Part print with two shaded views. Sizes in mm from the minimum x, y, z corner. Coordinates: 2 decimals unless noted, no trailing zeros. Loops run counter-clockwise (first coordinate to the right, second up) from the corner with the lowest first, then second, coordinate; pieces in that order, holes last. Notation, with made-up numbers: (49, 29) -> (97, 29) arc R22 cw to (97, 52) -> close; hole circle Ø1 at (71, 9.25). An arc over 180 degrees is marked (long way). Use one line per item in the form item = value.
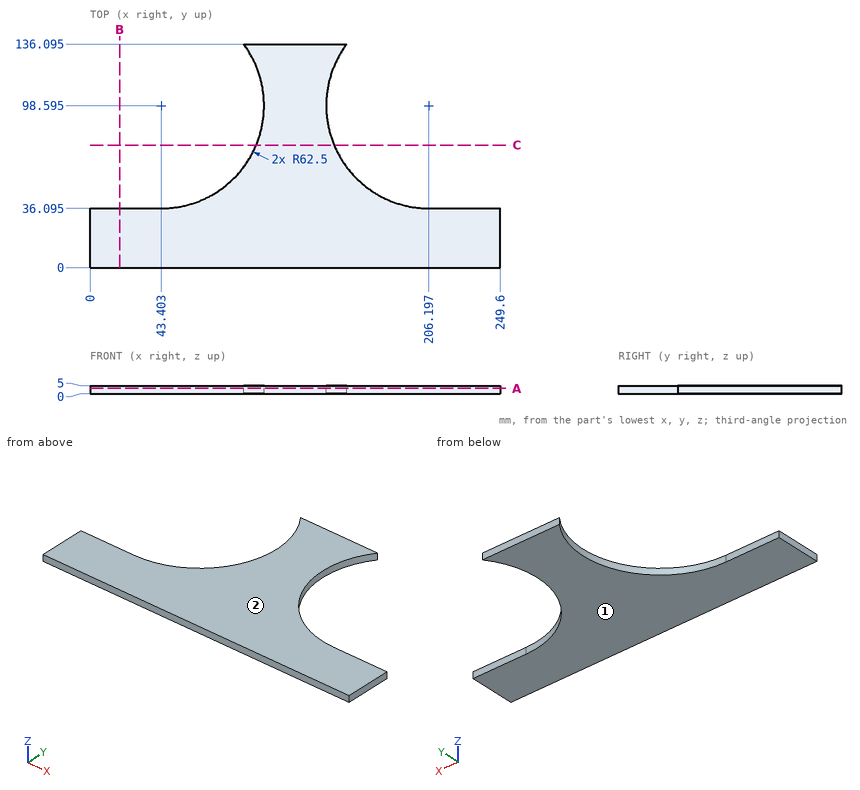
Q1. Band-saw the part on A-A, the plane z = 3.4. Write the cut outline in (x, y) (1 decimal).
Result:
outline = (0, 0) -> (249.6, 0) -> (249.6, 36.1) -> (206.2, 36.1) arc R62.5 cw to (156.2, 136.1) -> (93.4, 136.1) arc R62.5 cw to (43.4, 36.1) -> (0, 36.1) -> close
Q2. Band-saw the part on B-B, the plane x = 18. Write the cut outline in (y, z) (1 decimal).
Result:
outline = (0, 0) -> (36.1, 0) -> (36.1, 5) -> (0, 5) -> close
Q3. Mould opens along Z. For the marked faces 1 and 2 say: released by +Z, released by -Z, zero draft, split by the parting line, or undercut.
Result:
face_1 = released by -Z
face_2 = released by +Z
Q4. Wall check: line 1 along X through (y, z) = (100, 2.2); line 2 along Y through (x, z) = (17, 1.85) (1 decimal); line 3 along Y through (x, z) = (193, 0.2) (1 decimal). Give the ranges that are in metal, low to high.
Result:
line_1 = 105.89 to 143.71
line_2 = 0 to 36.1
line_3 = 0 to 37.5
Q5. Band-saw the part on C-C, the plane y = 74.5. Write the cut outline in (x, z), and give its area (3 significant figures).
Result:
outline = (101.07, 0) -> (148.53, 0) -> (148.53, 5) -> (101.07, 5) -> close
area = 237 mm2
Q6. Pin check, flat tips, straight feed: pin 1 Ø1 at (y, z) = (57.5, 1.5) entering from -X; pin 2 Ø1.5 at (x, z) = (224.5, 1.5) entering from +Y (1 decimal); pin 3 Ø4 at (x, y) = (51, 15) entering from -Z. Stop position of each tip, or through.
Result:
pin_1 = 90.05
pin_2 = 36.1
pin_3 = 0
